Here's the drawing with two shaded views (mm, measured from the low corner). I have some questions. Coordinates: 2 decimals unless noted, no trailing zeros. Order: outer loops, then holes, each group sorted by start corner. A loop starts at its lowest first (then second) coordinate and runs counter-clockwise, first axis right, second up. Notation, with made-up numbers: (13.25, 68.25) -> (28.25, 68.25) arc R22 ccw to (28.25, 98.25) -> close; hole circle Ø1 at (-12, 65). An arc over 180 degrees is marked (long way). Answer in a Markdown table with one row per item. Add a question column.
1. Imagine slicing it at B-B on y = 16.5. Write out the boundary of the cut face in (x, z).
2. If I drill on line 1 along Z through (x, y) = (0.75, 21); line 2 along Y through (x, z) = (0.7, 21); line 3 along Z through (x, y) = (1.65, 20), over which ranges is the centre line in solid material (lowest first)? Write a range as [from, to].
3. Imagine slicing it at D-D on y = 26. Write out the boundary of the cut face in (x, z), plus the area to 3 significant figures.
4. Imagine slicing it at C-C on x = 0.6. Write out the boundary of the cut face in (y, z), plus the area to 3 significant figures.
5. Imagine slicing it at A-A on z = 92. Write out the boundary of the cut face in (x, y).
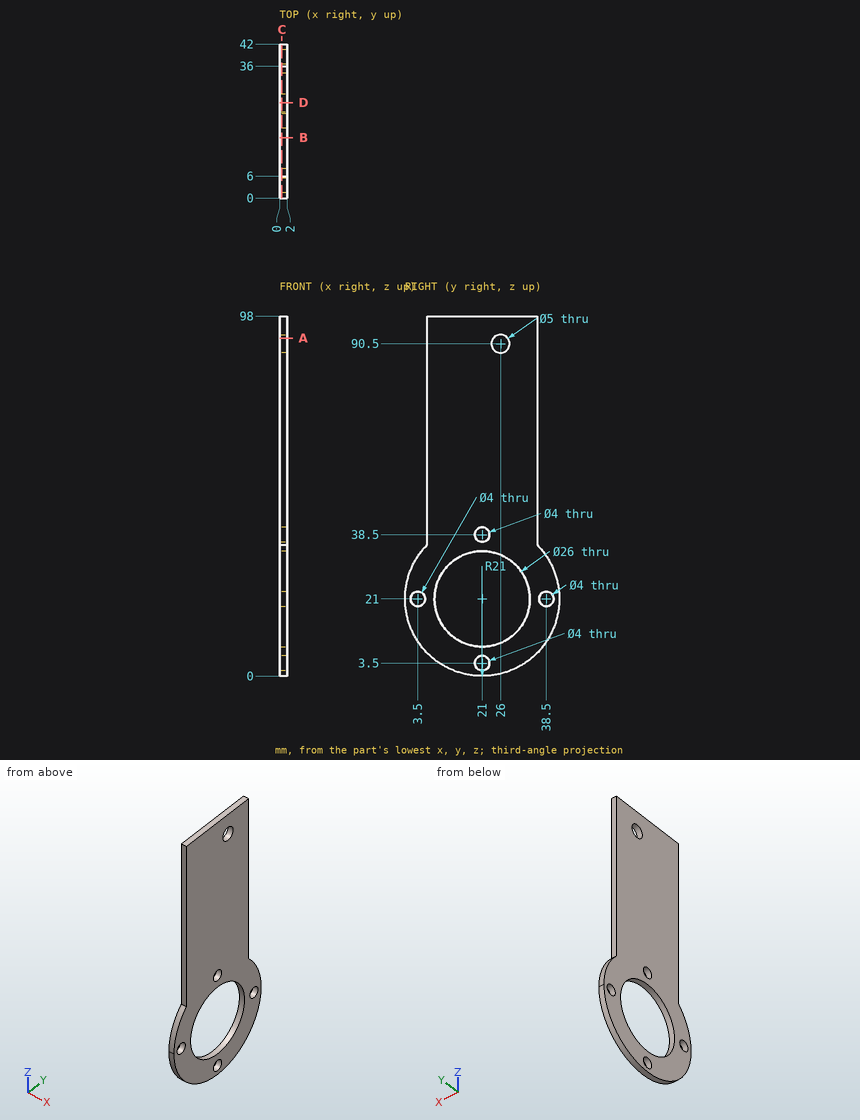
Answers follow:
| question | item | result |
|---|---|---|
| 1 | outline | (0, 0.49) -> (2, 0.49) -> (2, 8.8) -> (0, 8.8) -> close; (0, 33.2) -> (2, 33.2) -> (2, 98) -> (0, 98) -> close |
| 2 | line 1 | z = [0, 1.5], [5.5, 8], [34, 36.5], [40.5, 98] |
| 2 | line 2 | y = [0, 1.5], [5.5, 8], [34, 36.5], [40.5, 42] |
| 2 | line 3 | z = [0.02, 1.77], [5.23, 8.04], [33.96, 36.77], [40.23, 98] |
| 3 | outline | (0, 0.6) -> (2, 0.6) -> (2, 9) -> (0, 9) -> close; (0, 33) -> (2, 33) -> (2, 88) -> (0, 88) -> close; (0, 93) -> (2, 93) -> (2, 98) -> (0, 98) -> close |
| 3 | area | 137 mm² |
| 4 | outline | (6, 35.7) arc R21 ccw (long way) to (36, 35.7) -> (36, 98) -> (6, 98) -> close; hole circle Ø4 at (3.5, 21); hole circle Ø26 at (21, 21); hole circle Ø4 at (21, 3.5); hole circle Ø4 at (21, 38.5); hole circle Ø5 at (26, 90.5); hole circle Ø4 at (38.5, 21) |
| 4 | area | 2,520 mm² |
| 5 | outline | (0, 6) -> (2, 6) -> (2, 24) -> (0, 24) -> close; (0, 28) -> (2, 28) -> (2, 36) -> (0, 36) -> close |
